from build123d import *

# Parameters (mm, degrees)
BOSS_EXTRUDE1_DEPTH     = 37
SKETCH2_W               = 5.5
SKETCH2_H               = 7.8
BOSS_EXTRUDE2_DEPTH     = 37
CUT_EXTRUDE1_DEPTH      = 89.460443137
CUT_EXTRUDE1_DEPTH_BACK = 89.460443137
SKETCH3_W               = 7.6
SKETCH3_H               = 17
CUT_EXTRUDE2_DEPTH      = 89.460443137
CUT_EXTRUDE2_DEPTH_BACK = 89.460443137
SKETCH4_R               = 1.2
CUT_EXTRUDE3_DEPTH      = 89.460443137
CUT_EXTRUDE3_DEPTH_BACK = 89.460443137
SKETCH5_W               = 2.5
SKETCH5_H               = 67
CUT_EXTRUDE4_DEPTH      = 90.09545443
CUT_EXTRUDE4_DEPTH_BACK = 10.5
SKETCH6_W               = 69.2
SKETCH6_H               = 61.2
SKETCH7_R               = 2.5
BOSS_EXTRUDE8_DEPTH     = 10.5
SKETCH8_R               = 1.3
CUT_EXTRUDE5_DEPTH      = 8
SKETCH9_R               = 1.5
CUT_EXTRUDE6_DEPTH      = 3


with BuildPart() as part:
    # Sketch1 → Boss-Extrude1 (new, symmetric)
    with BuildSketch(Plane.XY):
        with BuildLine():
            Line((7.5, 0), (7.5, -80))
            Line((7.5, -80), (-7.5, -80))
            Line((-7.5, -80), (-7.5, 0))
            ThreePointArc((-7.5, 0), (0, 7.5), (7.5, 0))
        make_face()
    extrude(amount=BOSS_EXTRUDE1_DEPTH, both=True)

    # Sketch2 → Boss-Extrude2 (add, symmetric)
    with BuildSketch(Plane.XY):
        with Locations((-4.75, 3.9)):
            Rectangle(SKETCH2_W, SKETCH2_H)
    extrude(amount=BOSS_EXTRUDE2_DEPTH, both=True)

    # Sketch3 → Cut-Extrude1 (cut, two sides: drawn at the far end of the back side and taken through both)
    with BuildSketch(Plane(origin=(0, 0, 0), x_dir=(0, 0, -1), z_dir=(1, 0, 0)).offset(-CUT_EXTRUDE1_DEPTH_BACK)):
        with Locations((-9.25, 0.5)):
            Rectangle(SKETCH3_W, SKETCH3_H)
        with Locations((-27.75, 0.5)):
            Rectangle(SKETCH3_W, SKETCH3_H)
        with Locations((27.75, 0.5)):
            Rectangle(SKETCH3_W, SKETCH3_H)
        with Locations((9.25, 0.5)):
            Rectangle(SKETCH3_W, SKETCH3_H)
    extrude(amount=CUT_EXTRUDE1_DEPTH + CUT_EXTRUDE1_DEPTH_BACK, mode=Mode.SUBTRACT)

    # Sketch4 → Cut-Extrude2 (cut, two sides: drawn at the far end of the back side and taken through both)
    with BuildSketch(Plane.XY.offset(-CUT_EXTRUDE2_DEPTH_BACK)):
        Circle(SKETCH4_R)
    extrude(amount=CUT_EXTRUDE2_DEPTH + CUT_EXTRUDE2_DEPTH_BACK, mode=Mode.SUBTRACT)

    # Sketch5 → Cut-Extrude3 (cut, two sides: drawn at the far end of the back side and taken through both)
    with BuildSketch(Plane.XY.offset(-CUT_EXTRUDE3_DEPTH_BACK)):
        with Locations((6.75, -47.5)):
            Rectangle(SKETCH5_W, SKETCH5_H)
    extrude(amount=CUT_EXTRUDE3_DEPTH + CUT_EXTRUDE3_DEPTH_BACK, mode=Mode.SUBTRACT)

    # Sketch6 → Cut-Extrude4 (cut, two sides: drawn at the far end of the back side and taken through both)
    with BuildSketch(Plane(origin=(5.5, 0, 0), x_dir=(0, 0, -1), z_dir=(1, 0, 0)).offset(-CUT_EXTRUDE4_DEPTH_BACK)):
        with Locations((0, -47)):
            Rectangle(SKETCH6_W, SKETCH6_H)
    extrude(amount=CUT_EXTRUDE4_DEPTH + CUT_EXTRUDE4_DEPTH_BACK, mode=Mode.SUBTRACT)

    # Sketch7 → Boss-Extrude8 (add)
    with BuildSketch(Plane(origin=(-5, 0, 0), x_dir=(0, 0, -1), z_dir=(1, 0, 0))):
        with Locations((-32.6, -69.6)):
            Circle(SKETCH7_R)
        with Locations((-32.6, -24.4)):
            Circle(SKETCH7_R)
        with Locations((32.6, -24.4)):
            Circle(SKETCH7_R)
        with Locations((32.6, -69.6)):
            Circle(SKETCH7_R)
    extrude(amount=BOSS_EXTRUDE8_DEPTH)

    # Sketch8 → Cut-Extrude5 (cut)
    with BuildSketch(Plane(origin=(5.5, 0, 0), x_dir=(0, 0, -1), z_dir=(1, 0, 0))):
        with Locations((-32.6, -24.4)):
            Circle(SKETCH8_R)
        with Locations((32.6, -24.4)):
            Circle(SKETCH8_R)
        with Locations((32.6, -69.6)):
            Circle(SKETCH8_R)
        with Locations((-32.6, -69.6)):
            Circle(SKETCH8_R)
    extrude(amount=-CUT_EXTRUDE5_DEPTH, mode=Mode.SUBTRACT)

    # Sketch9 → Cut-Extrude6 (cut)
    with BuildSketch(Plane.XZ.offset(80)):
        with Locations(Location((0, -9.25, 0), (0, 0, 270))):
            Circle(SKETCH9_R)
        with Locations(Location((0, -27.75, 0), (0, 0, 270))):
            Circle(SKETCH9_R)
        with Locations(Location((0, 9.25, 0), (0, 0, 270))):
            Circle(SKETCH9_R)
        with Locations(Location((0, 27.75, 0), (0, 0, 270))):
            Circle(SKETCH9_R)
    extrude(amount=-CUT_EXTRUDE6_DEPTH, mode=Mode.SUBTRACT)


solid = part.part
The listing builds one solid part. Answer for the finished solid, in the listing's coordinates (mm). A direction names the side the tool comes from. Round coordinates to 2 decimals unless told otherwise and drop trailing zeros. Write each loop counter-clockwise with the first axis right and the second up, starting at its lowest first coordinate (ties: lowest second). Pieces come first, ordered by that corner, then holes. Notation, with made-up numbers: M -4.75,84 L 16.25,84 A7 cw 16.25,94 Z; hole C -31.75,-33 d4. An arc over 180 degrees is marked long. Write each question's results on one line, items separated by ' | '. Start each with the question number.
(1) The part is cut by section A-A, the plane y = -4. Write down the section's boundary in (x, z), and give its area (3 significant figures).
(2) The part is cut by section B-B, the plane z = -16. Write down the section's boundary in (x, y).
(3) Each of these flat-tipped pins is pushed along its axis until it touches: P1, Ø0.8, axis at y = -24, z = 32.5, coming from the +X side; P2, Ø2.5, axis at x = -2.5, z = 7.5, coming from the +Y side; P3, Ø6, axis at y = -40, z = -19.5, coming from the +X side. Where does it stop, or does it pass through?
(4) Determine the mould class of faces 5 (the flat face through (-5, 7.8, 19)), 6 (the flat face through (-5, -47, 0)), 7 (the flat face through (-2, 0, 13.05)) for opening direction Y: +Y half, -Y half, draft (parallel to the pull), parting line (faces both ways), or undercut.
(5) The part is cut by section C-C, the plane z = -27.75. Write down the section's boundary in (x, y), and give its area (3 significant figures).
(6) Find the intervals of material crossed by line 1 (Z direction, x = -2, y = 0); line 2 (Z direction, x = 1, y = -69.6); line 3 (Y direction, x = 4.5, z = 25), in increasing order.
(7) The part is cut by section D-D, the plane x = -6. Write down the section's boundary in (y, z).
(8) For faces 1 (the flat face through (-1, -80, 1)), 2 (the flat face through (5.5, -15, 0)), 3 (the flat face through (0, -47, 34.6)), 4 (the flat face through (-2, 0, 5.45)), determine the directions among +Z, -Z, +X, -X, +Y, -Y from which every point of the face is accessible in a straight line to the end or side of a thin tool.
Worked answers:
1) outline: M -7.5,-37 L 7.5,-37 L 7.5,-31.55 L -7.5,-31.55 Z; M -7.5,-23.95 L 7.5,-23.95 L 7.5,-13.05 L -7.5,-13.05 Z; M -7.5,-5.45 L 7.5,-5.45 L 7.5,5.45 L -7.5,5.45 Z; M -7.5,13.05 L 7.5,13.05 L 7.5,23.95 L -7.5,23.95 Z; M -7.5,31.55 L 7.5,31.55 L 7.5,37 L -7.5,37 Z | area: 654 mm²
2) outline: M -7.5,-80 L 5.5,-80 L 5.5,-77.6 L -5,-77.6 L -5,-16.4 L 5.5,-16.4 L 5.5,-14 L 7.5,-14 L 7.5,0 A7.5 ccw -2,7.23 L -2,7.8 L -7.5,7.8 Z; hole C 0,0 d2.4
3) P1: stops at x = -2.5 | P2: stops at y = -8 | P3: stops at x = -5
4) face 5: +Y half | face 6: undercut | face 7: draft
5) outline: M -7.5,-80 L -1.5,-80 L -1.5,-77.6 L -5,-77.6 L -5,-16.4 L 5.5,-16.4 L 5.5,-14 L 7.5,-14 L 7.5,-8 L -7.5,-8 Z; M 1.5,-80 L 5.5,-80 L 5.5,-77.6 L 1.5,-77.6 Z | area: 298 mm²
6) line 1: z = -37 to -31.55, -23.95 to -13.05, -5.45 to 5.45, 13.05 to 23.95, 31.55 to 37 | line 2: z = -37 to -33.9, -31.3 to -30.1, 30.1 to 31.3, 33.9 to 37 | line 3: y = -80 to -77.6, -16.4 to -8
7) outline: M -80,-37 L 7.8,-37 L 7.8,-31.55 L -8,-31.55 L -8,-23.95 L 7.8,-23.95 L 7.8,-13.05 L -8,-13.05 L -8,-5.45 L 7.8,-5.45 L 7.8,5.45 L -8,5.45 L -8,13.05 L 7.8,13.05 L 7.8,23.95 L -8,23.95 L -8,31.55 L 7.8,31.55 L 7.8,37 L -80,37 Z
8) face 1: +Z, -Z, +X, -X, -Y | face 2: +Z, -Z, +X, -Y | face 3: +X | face 4: +X, -X, +Y
